CAD build for the part. Positions are in the model's coordinates, mm. Face numbers are marked on the shaded views. A direction names the side the tool comes from. Give positions to 0.01 mm unless a question says otherwise; leave off trailing zeros. Loops run counter-clockwise (first coordinate to the right, second up) from the corner with the lowest first, then second, coordinate; pieces in that order, holes last.
Item 1: Saw through at C-C on z = -2.5. Give the cut face in (x, y), plus the area to 3 significant figures.
Item 2: Drop flat-ended pins along their axis: P1, Ø2, axis at y = 12.5, z = 1.5, coming from the +X side; P2, Ø11, axis at x = 14.5, y = 12, coming from the -Z side; P3, Ø8, axis at x = -16, z = -4, coming from the +Y side. Give the stop position or say it passes through.
Item 3: Probe probe 1 along Y at (x, z) = (-18.5, 8); probe 2 along X at (y, z) = (7.5, -3.5); probe 3 along Z at (x, y) = (-0.5, -3.5). List the from-to ranges inside material, lowest first.
Item 4: Saw through at B-B on x = 15.5. Give the cut face in (y, z).
Item 5: Saw through at D-D on y = 3.75. Give the cut face in (x, z).
Item 6: Which spindle directions (+Z, -Z, +X, -X, +Y, -Y) get a long thin tool onto all of the face, cutting with end or side? Do the marked faces 4, 5, 6 and 7. Say none if no direction does.
Item 7: Saw through at A-A on y = -5.25. Give the cut face in (x, z), plus the area to 3 significant figures.
Item 8: Mould opens along Z. For the marked faces 1, 2 and 3 say: released by +Z, released by -Z, zero draft, split by the parting line, or undercut.
from build123d import *

# Parameters (mm, degrees)
F0_W     = 45
F0_H     = 20
F1_DEPTH = 7
F3_DEPTH = 5
F4_W     = 10
F4_H     = 6
F5_DEPTH = 25


with BuildPart() as f1:
    # F0 (on Front) → F1 (new body)
    with BuildSketch(Plane.XZ):
        with Locations((0.659725, 0.518122)):
            Rectangle(F0_W, F0_H)
    extrude(amount=F1_DEPTH)

    # F2 (on face) → F3 (cut)
    with BuildSketch(Plane.XZ.offset(7)):
        Polygon((-2.808699, 4.728764), (-5.499579, -0.068023), (-2.69088, -4.796787), (2.808699, -4.728764), (5.499579, 0.068023), (2.69088, 4.796787), align=None)
    extrude(amount=-F3_DEPTH, mode=Mode.SUBTRACT)

    # F4 (on face) → F5 (join)
    with BuildSketch(Plane.XZ.offset(7)):
        with Locations((14.343088, -0.862489)):
            Rectangle(F4_W, F4_H)
    extrude(amount=-F5_DEPTH)


solid = f1.part
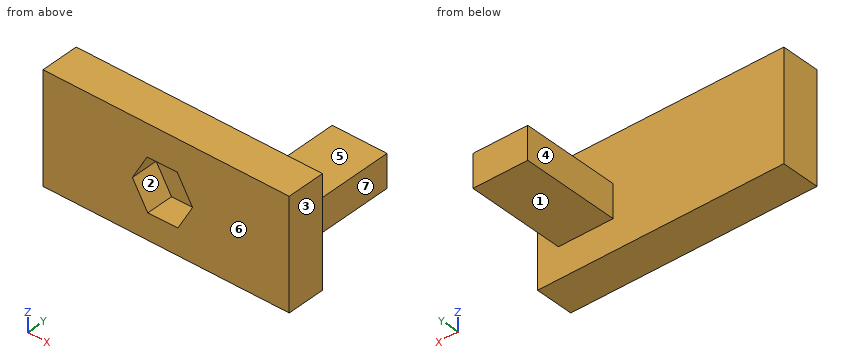
Results below:
1. outline: (-21.84, -7) - (-4.06, -7) - (-4.06, -2) - (4.06, -2) - (4.06, -7) - (23.16, -7) - (23.16, 0) - (19.34, 0) - (19.34, 18) - (9.34, 18) - (9.34, 0) - (-21.84, 0) - close
1. area: 454 mm2
2. P1: stops at x = 19.34
2. P2: stops at z = -3.86
2. P3: stops at y = 0
3. probe 1: y = -7 to 0
3. probe 2: x = 9.34 to 19.34
3. probe 3: z = -9.48 to -4.77, 4.76 to 10.52
4. outline: (-7, -9.48) - (0, -9.48) - (0, -3.86) - (18, -3.86) - (18, 2.14) - (0, 2.14) - (0, 10.52) - (-7, 10.52) - close
5. outline: (9.34, -3.86) - (19.34, -3.86) - (19.34, 2.14) - (9.34, 2.14) - close
6. face 4: +Z, -Z, -X, +Y
6. face 5: +Z, +X, -X, +Y
6. face 6: +Z, -Z, +X, -X, -Y
6. face 7: +Z, -Z, +X, +Y
7. outline: (-21.84, -9.48) - (23.16, -9.48) - (23.16, 10.52) - (-21.84, 10.52) - close; hole (-5.5, -0.07) - (-2.69, -4.8) - (2.81, -4.73) - (5.5, 0.07) - (2.69, 4.8) - (-2.81, 4.73) - close
7. area: 821 mm2
8. face 1: released by -Z
8. face 2: undercut
8. face 3: zero draft
